```python
from build123d import *

# Parameters (mm, degrees)
CONG_1_R                 = 0.2
CONG_2_R                 = 0.2
CHANFREIN1_SIZE          = 0.7
CHANFREIN1_SIZE2         = 0.454585315
CONG_3_R                 = 2
ESQUISSE2_W              = 0.4
ESQUISSE2_H              = 2.6
BOSS_EXTRU_1_DEPTH       = 6
ESQUISSE3_R              = 0.64
ENL_V_MAT_EXTRU_1_DEPTH  = 6
CONG_4_R                 = 1
RESSALTO_EXTRUS_O1_DEPTH = 0.5


with BuildPart() as part:
    # Esquisse1 → Révolution1 (revolve)
    with BuildSketch(Plane.XY, mode=Mode.PRIVATE) as r_volution1_sk:
        with BuildLine():
            Line((0, 18.8), (0, 0))
            Line((0, 0), (3.69, 0))
            Line((3.69, 0), (3.69, 7))
            Line((3.69, 7), (4.84, 7))
            Line((4.84, 7), (4.84, 15))
            Line((4.84, 15), (6.01, 15))
            Line((6.01, 15), (6.01, 16))
            ThreePointArc((6.01, 16), (5.013982948, 16.330092875), (4, 16.6))
            Line((4, 16.6), (4, 15.013190638))
            Line((4, 15.013190638), (3.89, 15.013190638))
            Line((3.89, 15.013190638), (3.89, 18.2))
            ThreePointArc((3.89, 18.2), (1.968000254, 18.649118314), (0, 18.8))
        make_face()
    revolve(r_volution1_sk.sketch.rotate(Axis((0, 0, 0), (0, 1, 0)), 90), axis=Axis((0, 0, 0), (0, 1, 0)))

    # Congé1
    cong_1_edges = [part.edges().sort_by_distance(p)[0] for p in [
        (0, 18.2, 3.89),
    ]]
    fillet(cong_1_edges, radius=CONG_1_R)

    # Congé2
    cong_2_edges = [part.edges().sort_by_distance(p)[0] for p in [
        (0, 16, 6.01),
    ]]
    fillet(cong_2_edges, radius=CONG_2_R)

    # Chanfrein1
    chanfrein1_edges = [part.edges().sort_by_distance(p)[0] for p in [
        (0, 7, 4.84),
    ]]
    chanfrein1_side = [part.faces().sort_by_distance(p)[0] for p in [
        (0, 11, 4.84),
    ]]
    chamfer(chanfrein1_edges, length=CHANFREIN1_SIZE, length2=CHANFREIN1_SIZE2, reference=chanfrein1_side[0])

    # Congé3
    cong_3_edges = [part.edges().sort_by_distance(p)[0] for p in [
        (0, 7.7, 4.84),
    ]]
    fillet(cong_3_edges, radius=CONG_3_R)

    # Esquisse2 → Boss.-Extru.1 (add)
    with BuildSketch(Plane.XZ):
        with Locations((2.3, 0)):
            Rectangle(ESQUISSE2_W, ESQUISSE2_H)
        with Locations((-2.3, 0)):
            Rectangle(ESQUISSE2_W, ESQUISSE2_H)
    extrude(amount=BOSS_EXTRU_1_DEPTH)

    # Esquisse3 → Enlèv. mat.-Extru.1 (cut)
    with BuildSketch(Plane.ZY.offset(2.5)):
        with Locations((0, -4.7)):
            Circle(ESQUISSE3_R)
        with BuildLine():
            Line((-1.3, -0.8), (-4.192462756, -0.8))
            Line((-4.192462756, -0.8), (-4.192462756, -7.475627282))
            Line((-4.192462756, -7.475627282), (5.572809524, -7.57510374))
            Line((5.572809524, -7.57510374), (5.225347222, -0.8))
            Line((5.225347222, -0.8), (1.3, -0.8))
            ThreePointArc((1.3, -0.8), (0.901580438, -2.499750503), (1.207561262, -4.218548238))
            ThreePointArc((1.207561262, -4.218548238), (0, -6), (-1.207561262, -4.218548238))
            ThreePointArc((-1.207561262, -4.218548238), (-0.901580438, -2.499750503), (-1.3, -0.8))
        make_face()
    extrude(amount=-ENL_V_MAT_EXTRU_1_DEPTH, mode=Mode.SUBTRACT)

    # Congé4
    cong_4_edges = [part.edges().sort_by_distance(p)[0] for p in [
        (-2.3, -0.8, 1.3),
        (-2.3, -0.8, -1.3),
        (2.3, -0.8, -1.3),
        (2.3, -0.8, 1.3),
    ]]
    fillet(cong_4_edges, radius=CONG_4_R)

    # Esboço1 → Ressalto-extrusão1 (add, symmetric)
    with BuildSketch(Plane(origin=(0, 18.243955153, 0), x_dir=(-1, 0, 0), z_dir=(0, -1, 0))):
        with BuildLine():
            Line((1.106856798, -0.603238885), (1.906856798, -0.603238885))
            ThreePointArc((1.906856798, -0.603238885), (-1.956724443, -0.413798809), (1.499383453, 1.323574426))
            Line((1.499383453, 1.323574426), (2.120884424, 1.323574426))
            ThreePointArc((2.120884424, 1.323574426), (-2.469207481, -0.39117057), (2.42612919, -0.603238885))
            Line((2.42612919, -0.603238885), (3.22612919, -0.603238885))
            Line((3.22612919, -0.603238885), (2.166492994, 0.456397311))
            Line((2.166492994, 0.456397311), (1.106856798, -0.603238885))
        make_face()
    extrude(amount=RESSALTO_EXTRUS_O1_DEPTH, both=True)


solid = part.part
```
Geometry check sheet. Reference: the model listing, model coordinates, mm. A direction names the side the tool comes from. Coordinates: 2 decimals unless noted, no trailing zeros. Order: outer loops, then holes, each group sorted by start corner. A loop starts at its lowest first (then second) coordinate and runs counter-clockwise, first axis right, second up. Notation, with made-up numbers: (27.5, -10) - (64.5, -10) arc R24 ccw to (64.5, 15) - close; hole circle Ø10 at (35, 61). An arc over 180 degrees is marked (long way). Answer as a JSON object with one key per item and string values. Group by question number.
Item 1: Draft check along Z on faces 6 (the face through (2.5, -3, 0)), 7 (the face through (-3.66, 3.55, 0.48)), 8 (the face through (2.297, -5.268, 0.295)). Enter one of: +Z half, -Z half, draft (parallel to the pull), parting line (faces both ways), or undercut.
Item 2: Tool access check on faces 1 (the face through (-2.5, -3, 0)), 2 (the face through (4.725, 11.693, 1.049)), 3 (the face through (-2, 18.744, 0)), 4 (the face through (-5.96, 15.44, 0.78)), 5 (the face through (-2.1, -3, 0)). Record the directions out of +Z, -Z, +X, -X, +Y, -Y that give a thin tool (end or side, any length) a straight path to the whole face; none if there is none.
Item 3: Sectioned sample at B-B, the plane y = -1.25. Record the cut outline in (x, z), and give its area (3 significant figures).
Item 4: Depth check by flat-ended pin: pin 1 Ø4 at (x, y) = (1.5, 3.5) entering from +Z; pin 2 Ø3 at (y, z) = (-2, -0.5) entering from +X; pin 3 Ø1 at (x, y) = (-3, 8) entering from -Z. Enter the tip coordinate at first touch or a pass-through.
Item 5: Scan lines: probe 1 along Y at (x, z) = (-2.3, 0); probe 2 along X at (y, z) = (-2.5, -0.25); probe 3 along X at (y, z) = (11, -1.75). Record each from-to range of solid material in increasing order.
Item 6: Sectioned sample at A-A, the plane y = -4.7. Record the cut outline in (x, z).
Item 7: Sectioned sample at C-C, the plane y = 6. Record the cut outline in (x, z).
Resolved:
{
 "1": {"face 6": "draft", "face 7": "parting line", "face 8": "undercut"},
 "2": {"face 1": "+Z, -Z, -X, -Y", "face 2": "-Y", "face 3": "+Y", "face 4": "+Y, -Y", "face 5": "+Z, -Z, -Y"},
 "3": {"outline": "(-2.5, -1.12) - (-2.1, -1.12) - (-2.1, 1.12) - (-2.5, 1.12) - close; (2.1, -1.12) - (2.5, -1.12) - (2.5, 1.12) - (2.1, 1.12) - close", "area": "1.79 mm^2"},
 "4": {"pin 1": "z = 3.69", "pin 2": "x = 2.5", "pin 3": "z = -4.13"},
 "5": {"probe 1": "-6 to -5.34, -4.06 to 18.74", "probe 2": "-2.5 to -2.1, 2.1 to 2.5", "probe 3": "-4.51 to 4.51"},
 "6": {"outline": "(-2.5, -1.3) - (-2.1, -1.3) - (-2.1, -0.64) - (-2.5, -0.64) - close; (-2.5, 0.64) - (-2.1, 0.64) - (-2.1, 1.3) - (-2.5, 1.3) - close; (2.1, -1.3) - (2.5, -1.3) - (2.5, -0.64) - (2.1, -0.64) - close; (2.1, 0.64) - (2.5, 0.64) - (2.5, 1.3) - (2.1, 1.3) - close"},
 "7": {"outline": "circle Ø7.38 at (0, 0)"}
}
